from build123d import *

# Parameters (mm, degrees)
SKETCH2_W                        = 30
SKETCH2_H                        = 15
BOSS_EXTRUDE1_DEPTH              = 10
BOUNDARY1_DEPTH                  = 30
BOSS_EXTRUDE2_DEPTH              = 30
SKETCH4_W                        = 30
SKETCH4_H                        = 15
BOSS_EXTRUDE3_DEPTH              = 100
SKETCH6_W                        = 18
SKETCH6_H                        = 15
BOSS_EXTRUDE4_DEPTH              = 9
BOSS_EXTRUDE5_DEPTH              = 18
CUT_EXTRUDE1_REACH               = 151.344
SKETCH8_R                        = 3
CUT_EXTRUDE2_REACH               = 139.38
SKETCH11_W                       = 30
SKETCH11_H                       = 15
SKETCH12_W                       = 30
SKETCH12_H                       = 15
BOSS_EXTRUDE7_DEPTH              = 50
BOSS_EXTRUDE8_DEPTH              = 30
SKETCH14_W                       = 30
SKETCH14_H                       = 15
BOSS_EXTRUDE10_DEPTH             = 20
BOSS_EXTRUDE11_DEPTH             = 30
SKETCH15_W                       = 5
SKETCH15_H                       = 15
BOSS_EXTRUDE12_DEPTH             = 7.5
SKETCH16_W                       = 5
SKETCH16_H                       = 7.5
REVOLVE1_ANGLE                   = 180
CUT_EXTRUDE3_REACH               = 202.419
SKETCH17_R                       = 3.175
SKETCH18_W                       = 4
SKETCH18_H                       = 25
CUT_EXTRUDE4_DEPTH               = 191.993712728
SKETCH20_R                       = 3.175
CUT_EXTRUDE5_DEPTH               = 201.546523118
SKETCH21_W                       = 30
SKETCH21_H                       = 12
BOSS_EXTRUDE13_DEPTH             = 5
BOSS_EXTRUDE13_DIRECTION_2_REACH = 203.104
SKETCH22_W                       = 30
SKETCH22_H                       = 2.975516747
BOSS_EXTRUDE14_DEPTH             = 5
BOSS_EXTRUDE14_DIRECTION_2_REACH = 203.104


# Read off the part's stored shape, not the designer's step: Boundary1
with BuildPart() as part:
    # Sketch2 → Boss-Extrude1 (new body)
    with BuildSketch(Plane.XY.offset(-30)):
        with Locations((15, 7.5)):
            Rectangle(SKETCH2_W, SKETCH2_H)
    extrude(amount=BOSS_EXTRUDE1_DEPTH)

    # Boundary1 outline → Boundary1 (add)
    with BuildSketch(Plane.YZ):
        Polygon((0, 0), (0, -20), (15, -20), (5, 0), align=None)
    extrude(amount=BOUNDARY1_DEPTH)

    # 3DSketch3 → Boss-Extrude2 (add)
    with BuildSketch(Plane(origin=(0, 15, -30), x_dir=(0, -1, 0), z_dir=(1, 0, 0))):
        Polygon((0, 0), (0.904610688, 5.13030215), (15, 0), align=None)
    extrude(amount=BOSS_EXTRUDE2_DEPTH)

    # Sketch4 → Boss-Extrude3 (add)
    with BuildSketch(Plane(origin=(0, -9.641814145, -26.490666647), x_dir=(1, 0, 0), z_dir=(0, 0.34202014332566943, 0.9396926207859081))):
        with Locations((15, 17.7606043)):
            Rectangle(SKETCH4_W, SKETCH4_H)
    extrude(amount=-BOSS_EXTRUDE3_DEPTH)

    # Sketch6 → Boss-Extrude4 (add)
    with BuildSketch(Plane(origin=(0, -43.843828478, -120.459928725), x_dir=(-1, 0, 0), z_dir=(0, -0.3420201433256693, -0.9396926207859083))):
        with Locations((-15, 17.7606043)):
            Rectangle(SKETCH6_W, SKETCH6_H)
    extrude(amount=BOSS_EXTRUDE4_DEPTH)

    # Sketch7 → Boss-Extrude5 (add)
    with BuildSketch(Plane.ZY.offset(-6)):
        with BuildLine():
            Line((-137.556797816, -23.184806311), (-132.426495666, -37.280195622))
            ThreePointArc((-132.426495666, -37.280195622), (-142.039341397, -32.797652042), (-137.556797816, -23.184806311))
        make_face()
    extrude(amount=-BOSS_EXTRUDE5_DEPTH)

    # Sketch8 → Cut-Extrude1 (cut, up to next)
    with BuildSketch(Plane.ZY.offset(-6), mode=Mode.PRIVATE) as cut_extrude1_sk1:
        with Locations((-134.991646741, -30.232500967)):
            Circle(SKETCH8_R)
    cut_extrude1_tool1 = extrude(cut_extrude1_sk1.sketch, amount=-CUT_EXTRUDE1_REACH, mode=Mode.PRIVATE) & part.part
    add(cut_extrude1_tool1.solids().sort_by_distance((6, -30.232501, -134.991647))[0], mode=Mode.SUBTRACT)

    # Sketch11 → Cut-Extrude2 (cut, up to next)
    with BuildSketch(Plane(origin=(0, -43.843828478, -120.459928725), x_dir=(-1, 0, 0), z_dir=(0, -0.3420201433256693, -0.9396926207859083)), mode=Mode.PRIVATE) as cut_extrude2_sk1:
        with Locations((-15, 17.7606043)):
            Rectangle(SKETCH11_W, SKETCH11_H)
    cut_extrude2_tool1 = extrude(cut_extrude2_sk1.sketch, amount=CUT_EXTRUDE2_REACH, mode=Mode.PRIVATE) & part.part
    add(cut_extrude2_tool1.solids().sort_by_distance((15, -27.15432, -126.534413))[0], mode=Mode.SUBTRACT)



with BuildPart() as body_2:
    # Sketch12 → Boss-Extrude7 (new body)
    with BuildSketch(Plane(origin=(0, -79.331775874, -45.802222156), x_dir=(1, 0, 0), z_dir=(0, -0.8660254037844397, -0.49999999999999833))):
        with Locations((15, -97.759523082)):
            Rectangle(SKETCH12_W, SKETCH12_H)
    extrude(amount=BOSS_EXTRUDE7_DEPTH)


with BuildPart() as part_1:
    add(part.part)

    add(body_2.part)  # Boss-Extrude8 merges body 2
    # 3DSketch4 → Boss-Extrude8 (add)
    with BuildSketch(Plane(origin=(0, -20.106625021, -129.099564228), x_dir=(0, -0.9396926207859082, 0.3420201433256692), z_dir=(1, 0, 0))):
        Polygon((0, 0), (3.509333353, 9.641814145), (15, 0), align=None)
    extrude(amount=BOSS_EXTRUDE8_DEPTH)



with BuildPart() as body_2_2:
    # Sketch14 → Boss-Extrude10 (new body)
    with BuildSketch(Plane(origin=(0, -77.503284522, 0), x_dir=(-1, 0, 0), z_dir=(0, -1, 0))):
        with Locations((-15, 156.469262079)):
            Rectangle(SKETCH14_W, SKETCH14_H)
    extrude(amount=BOSS_EXTRUDE10_DEPTH)


with BuildPart() as part_2:
    add(part_1.part)

    add(body_2_2.part)  # Boss-Extrude11 merges body 2 2
    # 3DSketch5 → Boss-Extrude11 (add)
    with BuildSketch(Plane(origin=(0, -77.503284522, -163.969262079), x_dir=(0, 0, 1), z_dir=(-1, 0, 0))):
        Polygon((0, 0), (15, 0), (2.009618943, 7.5), align=None)
    extrude(amount=-BOSS_EXTRUDE11_DEPTH)

    # Sketch15 → Boss-Extrude12 (add)
    with BuildSketch(Plane.XZ.offset(97.503284522)):
        with Locations((7.5, -156.469262079)):
            Rectangle(SKETCH15_W, SKETCH15_H)
        with Locations((22.5, -156.469262079)):
            Rectangle(SKETCH15_W, SKETCH15_H)
    extrude(amount=BOSS_EXTRUDE12_DEPTH)

    # Sketch16 → Revolve1 (revolve)
    with BuildSketch(Plane.XZ.offset(105.003284522)):
        with Locations((22.5, -160.219262079)):
            Rectangle(SKETCH16_W, SKETCH16_H)
        with Locations((7.5, -160.219262079)):
            Rectangle(SKETCH16_W, SKETCH16_H)
    revolve(axis=Axis((25, -105.003284522, -156.469262079), (-1, 0, 0)), revolution_arc=REVOLVE1_ANGLE)

    # Cut-Extrude3: up to this face of the body (flat: up to its plane)
    cut_extrude3_end = Plane(part_2.part.faces().sort_by_distance((25, -104.30316058, -156.469262079))[0])
    # Sketch17 → Cut-Extrude3 (cut, up to the picked face)
    with BuildSketch(Plane.ZY.offset(-5), mode=Mode.PRIVATE) as cut_extrude3_sk1:
        with Locations((-156.469262079, -105.003284522)):
            Circle(SKETCH17_R)
    cut_extrude3_tool1 = split(extrude(cut_extrude3_sk1.sketch, amount=-CUT_EXTRUDE3_REACH, mode=Mode.PRIVATE), bisect_by=cut_extrude3_end, keep=Keep.BOTH, mode=Mode.PRIVATE)
    add(cut_extrude3_tool1.solids().sort_by(Axis((5, -105.003285, -156.469262), (1, 0, 0)))[0], mode=Mode.SUBTRACT)

    # Sketch18 → Cut-Extrude4 (cut, through all)
    with BuildSketch(Plane(origin=(0, 52.629761541, -91.157420979), x_dir=(-1, 0, 0), z_dir=(0, 0.4999999999999983, -0.8660254037844398))):
        with Locations((-2, -129.104444312)):
            Rectangle(SKETCH18_W, SKETCH18_H)
        with Locations((-28, -129.104444312)):
            Rectangle(SKETCH18_W, SKETCH18_H)
    extrude(amount=-CUT_EXTRUDE4_DEPTH, mode=Mode.SUBTRACT)

    # Sketch20 → Cut-Extrude5 (cut, through all)
    with BuildSketch(Plane.ZY.offset(-4)):
        with Locations((-149.214452607, -62.927966974)):
            Circle(SKETCH20_R)
    extrude(amount=-CUT_EXTRUDE5_DEPTH, mode=Mode.SUBTRACT)

    # Sketch21 → Boss-Extrude13 (add)
    with BuildSketch(Plane(origin=(0, 0, 0), x_dir=(-1, 0, 0), z_dir=(0, -0.8036491793257791, 0.5951033494856183))):
        with Locations((-15, 6)):
            Rectangle(SKETCH21_W, SKETCH21_H)
    extrude(amount=BOSS_EXTRUDE13_DEPTH)

    # Sketch21 → Boss-Extrude13 direction 2 (add, up to next)
    with BuildSketch(Plane(origin=(0, 0, 0), x_dir=(-1, 0, 0), z_dir=(0, -0.8036491793257791, 0.5951033494856183)), mode=Mode.PRIVATE) as boss_extrude13_direction_2_sk1:
        with Locations((-15, 6)):
            Rectangle(SKETCH21_W, SKETCH21_H)
    boss_extrude13_direction_2_tool1 = extrude(boss_extrude13_direction_2_sk1.sketch, amount=-BOSS_EXTRUDE13_DIRECTION_2_REACH, mode=Mode.PRIVATE) - part_2.part
    add(boss_extrude13_direction_2_tool1.solids().sort_by_distance((15, -3.57062, -4.821895))[0])

    # Sketch22 → Boss-Extrude14 (add)
    with BuildSketch(Plane(origin=(0, 0, 0), x_dir=(-1, 0, 0), z_dir=(0, -0.8036491793257791, 0.5951033494856183))):
        with Locations((-15, -1.487758374)):
            Rectangle(SKETCH22_W, SKETCH22_H)
    extrude(amount=BOSS_EXTRUDE14_DEPTH)

    # Boss-Extrude14 direction 2: up to this plane
    boss_extrude14_direction_2_end = Plane(origin=(0, 5, 0), z_dir=(0, 0.894427190999916, 0.447213595499958))
    # Sketch22 → Boss-Extrude14 direction 2 (add, up to the surface)
    with BuildSketch(Plane(origin=(0, 0, 0), x_dir=(-1, 0, 0), z_dir=(0, -0.8036491793257791, 0.5951033494856183)), mode=Mode.PRIVATE) as boss_extrude14_direction_2_sk1:
        with Locations((-15, -1.487758374)):
            Rectangle(SKETCH22_W, SKETCH22_H)
    boss_extrude14_direction_2_tool1 = split(extrude(boss_extrude14_direction_2_sk1.sketch, amount=-BOSS_EXTRUDE14_DIRECTION_2_REACH, mode=Mode.PRIVATE), bisect_by=boss_extrude14_direction_2_end, keep=Keep.BOTH, mode=Mode.PRIVATE)
    add(boss_extrude14_direction_2_tool1.solids().sort_by_distance((15, 0.88537, 1.195636))[0])


solid = part_2.part
Could you check a few things on this model? Use its own coordinates, in mm. A direction names the side the tool comes from. Give positions to 0.01 mm unless a question says otherwise; leave off trailing zeros. Order: outer loops, then holes, each group sorted by start corner. A loop starts at its lowest first (then second) coordinate and runs counter-clockwise, first axis right, second up.
1. Suppose I cut it at A-A (y = -4). Write out the boundary of the cut face in (x, z).
Answers below:
outline: (0, -84.85) - (30, -84.85) - (30, -40.99) - (0, -40.99) - close; (0, -11.97) - (30, -11.97) - (30, 3) - (0, 3) - close
2. Which directions (+Z, -Z, +X, -X, +Y, -Y) give clear straight access to the entire face, cutting with the end or side of a thin tool? Please do faces 4 (the flat face through (26, -66.3, -149.3)), 5 (the flat face through (15.21, -5.66, -10.74)), 6 (the flat face through (15, -88, -148.969)).
Answers below:
face 4: +X
face 5: +X, -X, -Y
face 6: +Z, +X, -X, -Y
3. Thinking about a two-plate mould opening in Z: for faces 1 (the flat face through (28, -97.503, -157)), 2 (the flat face through (15, 0, -22)), 3 (the cylindrical face through (22.54, -112.5, -156.63)), which applies, +Z half, -Z half, draft (parallel to the pull), parting line (faces both ways), or undercut?
Answers below:
face 1: draft
face 2: undercut
face 3: parting line
4. For pin 1 (5 mm diameter, centred on x = 12.5, y = -56.5, fed in from -Z); pin 2 (5 mm diameter, centred on y = -62.93, z = -149.21, fed in from +X); pin 3 (8 mm diameter, centred on x = 15.5, z = -160, fed in from -Y); pin 4 (8.5 mm diameter, centred on y = -105, z = -156.47, fed in from +X), each with a flat end and sliding along its axis, tell me the tip position at first contact or that it passes through.
Answers below:
pin 1: stops at z = -155.61
pin 2: passes through
pin 3: stops at y = -97.5
pin 4: stops at x = 25
5. Suppose I cut it at C-C (z = -116). Write out the boundary of the cut face in (x, y).
Answers below:
outline: (0, -31.3) - (30, -31.3) - (30, -15.34) - (0, -15.34) - close
6. I need wall thicknesses on L1, parallel to Z at x = 28.75, y = -88; L2, parallel to Y at x = 15, z = -23; L3, parallel to Y at x = 5.75, z = -147.5. Which ranges of each line are inside material? Lowest first, please.
Answers below:
L1: z = -163.97 to -148.97
L2: y = 0 to 15
L3: y = -74.96 to -65.6, -60.26 to -44.96
7. Suppose I cut it at D-D (y = -85). Write out the boundary of the cut face in (x, z), plus the area to 3 significant figures.
Answers below:
outline: (0, -163.97) - (30, -163.97) - (30, -148.97) - (0, -148.97) - close
area: 450 mm2
